Geometry check sheet. Reference: the model listing, model coordinates, mm. Give positions to 0.01 mm unless a question says otherwise; leave off trailing zeros. Loops run counter-clockwise (first coordinate to the right, second up) from the corner with the lowest first, then second, coordinate; pieces in that order, holes last.
```python
from build123d import *

# Parameters (mm, degrees)
SKETCH1_W           = 130
SKETCH1_H           = 50
BOSS_EXTRUDE1_DEPTH = 5
FILLET1_R           = 5
SKETCH2_W           = 87.3
SKETCH2_H           = 41.7
CUT_EXTRUDE1_DEPTH  = 5


with BuildPart() as part:
    # Sketch1 → Boss-Extrude1 (new body)
    with BuildSketch(Plane.XY):
        Rectangle(SKETCH1_W, SKETCH1_H)
    extrude(amount=BOSS_EXTRUDE1_DEPTH)

    # Fillet1
    fillet1_edges = [part.edges().sort_by_distance(p)[0] for p in [
        (-65, 25, 2.5),
        (65, 25, 2.5),
    ]]
    fillet(fillet1_edges, radius=FILLET1_R)

    # Sketch2 → Cut-Extrude1 (cut)
    with BuildSketch(Plane.XY.offset(5)):
        Rectangle(SKETCH2_W, SKETCH2_H)
    extrude(amount=-CUT_EXTRUDE1_DEPTH, mode=Mode.SUBTRACT)


solid = part.part
```
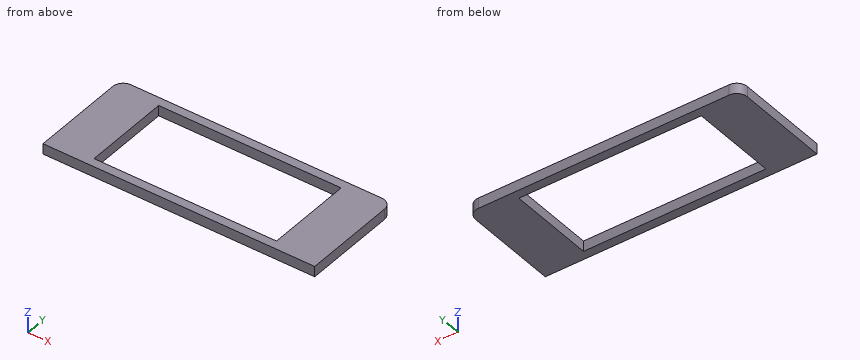
1) Sectioned sample at B-B on z = 3.25. Enter the section's corners in (x, y), plus the area to 3 significant figures.
2) Scan lines: line 1 along X through (y, z) = (-10, 2.9); line 2 along Y through (x, z) = (-8.5, 4.1); line 3 along X through (y, z) = (21, 3.3). Record each from-to range of solid material in increasing order.
3) Sectioned sample at C-C on y = -8. Enter the section's corners in (x, z), plus the area to 4 significant figures.
4) Sectioned sample at A-A on x = -36.5. Enter the section's corners in (y, z).
Determined:
1. outline: (-65, -25) - (65, -25) - (65, 20) arc R5 ccw to (60, 25) - (-60, 25) arc R5 ccw to (-65, 20) - close; hole (-43.65, -20.85) - (43.65, -20.85) - (43.65, 20.85) - (-43.65, 20.85) - close
1. area: 2,850 mm2
2. line 1: x = -65 to -43.65, 43.65 to 65
2. line 2: y = -25 to -20.85, 20.85 to 25
2. line 3: x = -64.9 to 64.9
3. outline: (-65, 0) - (-43.65, 0) - (-43.65, 5) - (-65, 5) - close; (43.65, 0) - (65, 0) - (65, 5) - (43.65, 5) - close
3. area: 213.5 mm2
4. outline: (-25, 0) - (-20.85, 0) - (-20.85, 5) - (-25, 5) - close; (20.85, 0) - (25, 0) - (25, 5) - (20.85, 5) - close
